Source: CAD feature listing. Evaluate the final solid. Frame: model axes, mm. Face numbers are marked on the shaded views. Coordinates: 2 decimals unless noted, no trailing zeros. Write each loop counter-clockwise with the first axis right and the second up, starting at its lowest first coordinate (ties: lowest second). Pieces come first, ordered by that corner, then holes. Notation, with made-up numbers: (33.25, -14.75) - (60.25, -14.75) arc R35 ccw to (60.25, 24.25) - close; hole circle Ø4 at (14.25, 8.25). An arc over 180 degrees is marked (long way). One line per question, with ' | ' between items.
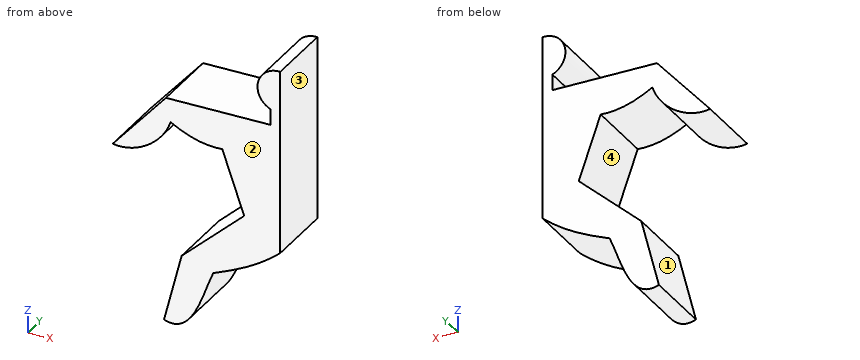
from build123d import *

# Parameters (mm, degrees)
F1_DEPTH = 25


with BuildPart() as f1:
    # F0 (on Front) → F1 (new body)
    with BuildSketch(Plane.XZ):
        with BuildLine():
            ThreePointArc((0, 44.947859), (-7.829862, 39.222287), (-3.407156, 30.589293))
            Line((-3.407156, 30.589293), (-3.407156, 24.967375))
            Line((-3.407156, 24.967375), (-40.440812, 24.967375))
            Line((-40.440812, 24.967375), (-59.282998, 3.510849))
            add(Edge.make_bspline(
                [(-59.282998, 3.510849), (-51.039223, 1.833404), (-41.357578, 8.351474), (-38.817345, 16.690769)],
                knots=[0, 0, 0, 0, 24.342418, 24.342418, 24.342418, 24.342418], degree=3))
            add(Edge.make_bspline(
                [(-38.817345, 16.690769), (-33.421371, 13.424438), (-26.868501, 11.176378), (-20.502377, 11.73953)],
                knots=[0, 0, 0, 0, 18.972422, 18.972422, 18.972422, 18.972422], degree=3))
            Line((-20.502377, 11.73953), (-12.747489, -10.253983))
            Line((-12.747489, -10.253983), (-34.881057, -30.43622))
            Line((-34.881057, -30.43622), (-41.132205, -55.052141))
            add(Edge.make_bspline(
                [(-41.132205, -55.052141), (-30.758676, -59.041798), (-27.452824, -41.829275), (-23.690994, -33.73597)],
                knots=[0, 0, 0, 0, 27.542239, 27.542239, 27.542239, 27.542239], degree=3))
            add(Edge.make_bspline(
                [(-23.690994, -33.73597), (-13.317464, -29.632323), (-6.705762, -26.098624), (0, -20.345102)],
                knots=[0, 0, 0, 0, 27.213573, 27.213573, 27.213573, 27.213573], degree=3))
            Line((0, -20.345102), (0, 44.947859))
        make_face()
    extrude(amount=F1_DEPTH)


solid = f1.part
Item 1: Pin query (flat end, axial travel): pin 1 Ø6 at (x, y) = (-49, -4.5) entering from -Z; pin 2 Ø6 at (x, y) = (-14.5, -15.5) entering from +Z; pin 3 Ø6 at (y, z) = (-8.5, 28.5) entering from -X. Return the tip coordinate at first contact, or that it passes through.
Check sheet entries:
pin 1: z = 3.95 | pin 2: z = 24.97 | pin 3: x = -5.02
Item 2: Mould query, pull axis X, two halves, no side actions, for the marked faces 1, 2, 3 and 4. Classes: pulls with the +X half, pulls with the -X half, needs draft (parallel to the pull), parting line crosses it, or undercut.
Check sheet entries:
face 1: pulls with the -X half | face 2: needs draft | face 3: pulls with the +X half | face 4: undercut
Item 3: Ray query, line 1 along X through (y, z) = (-9.75, 8); line 2 along X through (y, z) = (-17.5, 14.5); line 3 along Z through (x, y) = (-7, -9.25). Return the intervals inside material, ascending. Write a range as [from, to].
Check sheet entries:
line 1: [-55.34, -44.7], [-19.18, 0] | line 2: [-49.63, -39.66], [-34.66, 0] | line 3: [-25.58, 24.97], [33.71, 41.29]
Item 4: Cut plane A-A on z = -15.5. Return loops of the section in (x, y), and give its area (3 significant figures).
Check sheet entries:
outline: (-18.5, -25) - (0, -25) - (0, 0) - (-18.5, 0) - close | area: 463 mm²
